Design review of the part built by this model. Coordinates are the model's own, in mm. A direction names the side the tool comes from. Give positions to 0.01 mm unless a question says otherwise; leave off trailing zeros. Order: outer loops, then holes, each group sorted by start corner. A loop starts at its lowest first (then second) coordinate and runs counter-clockwise, first axis right, second up. Notation, with made-up numbers: (31, 71.5) -> (46, 71.5) arc R17 cw to (46, 102.5) -> close; hole circle Ø4 at (21.5, 31). An arc over 180 degrees is marked (long way). Use a Markdown table: item, result. Add a question column.
```python
from build123d import *

# Parameters (mm, degrees)
SKETCH1_W           = 45
SKETCH1_H           = 40
BOSS_EXTRUDE1_DEPTH = 6
SKETCH2_W           = 5
SKETCH2_H           = 5
SKETCH2_W_2         = 3.698246201
SKETCH2_H_2         = 10
SKETCH2_H_3         = 3
CUT_EXTRUDE1_DEPTH  = 6
SKETCH3_W           = 5
SKETCH3_H           = 5
CUT_EXTRUDE2_DEPTH  = 6
SKETCH4_W           = 5
SKETCH4_H           = 4.992810735
SKETCH4_H_2         = 10
SKETCH4_H_3         = 3
CUT_EXTRUDE3_DEPTH  = 6


with BuildPart() as part:
    # Sketch1 → Boss-Extrude1 (new body)
    with BuildSketch(Plane.XY):
        with Locations((8.087316256, -14.086161404)):
            Rectangle(SKETCH1_W, SKETCH1_H)
    extrude(amount=BOSS_EXTRUDE1_DEPTH)

    # Sketch2 → Cut-Extrude1 (cut)
    with BuildSketch(Plane.XY.offset(6)):
        with Locations((-11.912683744, -6.586161404)):
            Rectangle(SKETCH2_W, SKETCH2_H)
        with Locations((-11.912683744, -16.586161404)):
            Rectangle(SKETCH2_W, SKETCH2_H)
        with Locations((-11.912683744, -26.586161404)):
            Rectangle(SKETCH2_W, SKETCH2_H)
        with Locations((28.738193155, 0.913838596)):
            Rectangle(SKETCH2_W_2, SKETCH2_H_2)
        with Locations((28.738193155, -11.586161404)):
            Rectangle(SKETCH2_W_2, SKETCH2_H)
        with Locations((28.738193155, -22.586161404)):
            Rectangle(SKETCH2_W_2, SKETCH2_H_3)
    extrude(amount=-CUT_EXTRUDE1_DEPTH, mode=Mode.SUBTRACT)

    # Sketch3 → Cut-Extrude2 (cut)
    with BuildSketch(Plane.XY.offset(6)):
        with Locations((28.087316256, -31.586161404)):
            Rectangle(SKETCH3_W, SKETCH3_H)
    extrude(amount=-CUT_EXTRUDE2_DEPTH, mode=Mode.SUBTRACT)

    # Sketch4 → Cut-Extrude3 (cut)
    with BuildSketch(Plane.XY.offset(6)):
        with Locations((28.087316256, -11.582566772)):
            Rectangle(SKETCH4_W, SKETCH4_H)
        with Locations((28.087316256, 0.913838596)):
            Rectangle(SKETCH4_W, SKETCH4_H_2)
        with Locations((28.087316256, -22.586161404)):
            Rectangle(SKETCH4_W, SKETCH4_H_3)
    extrude(amount=-CUT_EXTRUDE3_DEPTH, mode=Mode.SUBTRACT)


solid = part.part
```
1) Insertion check: pin 1 (1.5 mm diameter, centred on x = 28.5, z = 2.5, fed in from -Y); pin 2 (1.5 mm diameter, centred on x = 29, z = 3.5, fed in from +Y); pin 3 (1.5 mm diameter, centred on y = -11.5, z = 2, fed in from +X). Each pin has a flat end and moves straight along its axis. Give the tip position at first contact, or say it passes through.
2) The part is to be moulded in two halves that separate along Y. For faces 4 (the flat face through (28, -4.086, 3)), 5 (the flat face through (-9.413, -17, 3)), 6 (the flat face through (8, -14, 0)), say which applies: +Y half, -Y half, draft (parallel to the pull), parting line (faces both ways), or undercut.
3) For L1, parallel to Y at x = 27, z = 3.3; L2, parallel to Y at x = -12, z = 1.65; L3, parallel to X at y = -3.5, z = 2.15, list the stretches that pass through material, from the lowest coordinate up. Write a range as [from, to].
4) Add section B-B (y = -8). Give the boundary of the cut face in (x, z).
5) Machinability: for faces 1 (the flat face through (-9.413, -27, 3)), 2 (the flat face through (28, -9.086, 3)), 3 (the flat face through (25.587, 1, 3)), which of the approach directions +Z, -Z, +X, -X, +Y, -Y give a long, thin tool a straight path to every point of the face, cutting with its end or side? Answer none if there is none.
Worked answers:
| question | item | result |
|---|---|---|
| 1 | pin 1 | y = -29.09 |
| 1 | pin 2 | y = -4.09 |
| 1 | pin 3 | x = 25.59 |
| 2 | face 4 | +Y half |
| 2 | face 5 | undercut |
| 2 | face 6 | draft |
| 3 | L1 | [-29.09, -24.09], [-21.09, -14.09], [-9.09, -4.09] |
| 3 | L2 | [-34.09, -29.09], [-24.09, -19.09], [-14.09, -9.09], [-4.09, 5.91] |
| 3 | L3 | [-14.41, 25.59] |
| 4 | outline | (-9.41, 0) -> (30.59, 0) -> (30.59, 6) -> (-9.41, 6) -> close |
| 5 | face 1 | +Z, -Z, -X |
| 5 | face 2 | +Z, -Z, +X |
| 5 | face 3 | +Z, -Z, +X, +Y |
